Could you check a few things on this model? Use its own coordinates, in mm. Give positions to 0.01 mm unless a question says otherwise; leave off trailing zeros. Loops run counter-clockwise (first coordinate to the right, second up) from the corner with the lowest first, then second, coordinate; pieces in that order, holes last. Notation, with made-up numbers: M 58,-29 L 93,-29 A20 ccw 93,10 Z; hole C 83.25,-13.75 d3. An arc over 180 degrees is marked long. Answer in a Markdown table with one row per item. Add a question column.
1. If we section it at B-B on z = 8: List the corners of the cut face in (x, y) for me.
2. I need wall thicknesses on line 1 along Y through (x, z) = (3.25, -14); line 2 along Y through (x, z) = (1.75, 40); line 3 along Z through (x, y) = (2.5, -50). Which ranges of each line are inside material? Lowest first, please. Write a range as from..to.
3. If we section it at A-A on y = -52: List the corners of the cut face in (x, z) for me, then the cut area to 3 significant figures.
4. If we section it at C-C on y = 33: List the corners of the cut face in (x, z) for me.
5. Thinking about a two-plate mould opening in Z: for faces 1 (the flat face through (10, -1, 1)), 2 (the flat face through (5, 1, 60)), 3 (the flat face through (2, -1, 0)), which applies, released by +Z, released by -Z, zero draft, split by the parting line, or undercut?
6. I'm going to push flat-ended pins straight in: pin 1 Ø8 at (y, z) = (-28, -11) entering from -X; pin 2 Ø1.5 at (y, z) = (61.25, 0) entering from -X. Where does each tip first touch, or does it pass through?
Autodesk Inventor part; units mm, degrees
ref_plane "YZ Plane" through (0, 0, 0) normal (1, 0, 0) x (0, 1, 0)
ref_plane "XZ Plane" through (0, 0, 0) normal (0, 1, 0) x (-1, 0, 0)
ref_plane "XY Plane" through (0, 0, 0) normal (0, 0, 1) x (1, 0, 0)
sketch "Boceto1" plane through (0, 0, 0) normal (1, 0, 0) x (0, 1, 0)
  line L0 (-57.5, -42.7876) -> (57.5, -42.7876)
  line L1 (57.5, -42.7876) -> (57.5, 42.2124)
  line L2 (57.5, 42.2124) -> (-57.5, 42.2124)
  line L3 (-57.5, 42.2124) -> (-57.5, -42.7876)
  line L4 (-57.5, -42.7876) -> (57.5, 42.2124) construction
  line L5 (57.5, -42.7876) -> (-57.5, 42.2124) construction
  point P0 (0, 0)
  point P1 (0, -0.2876)
  dimension "d0" = 115
  dimension "d1" = 85
sketch "Boceto2" plane through (0, 0, 0) normal (1, 0, 0) x (0, 1, 0)
  line L0 (-65, -60) -> (65, -60)
  line L1 (65, -60) -> (65, 60)
  line L2 (65, 60) -> (-65, 60)
  line L3 (-65, 60) -> (-65, -60)
  line L4 (-65, -60) -> (65, 60) construction
  line L5 (65, -60) -> (-65, 60) construction
  point P0 (0, 0)
  dimension "d2" = 130
  dimension "d3" = 120
extrude "Extrusión1" add sketch "Boceto2" along normal blind 10
extrude "Extrusión2" cut sketch "Boceto1" along normal blind 2
sketch "Boceto3" plane through (0, 0, 0) normal (-1, 0, 0) x (0, 0, 1)
  line L0 (0, 0) -> (0, -52)
  line L1 (0, 0) -> (0, 52)
  line L2 (-60, -65) -> (-60, 65)
  line L3 (0, -52) -> (46, -52)
  line L4 (0, -52) -> (-46, -52)
  line L5 (-46, -52) -> (-48.5, -52)
  circle A0 centre (-48.5, -52) radius 2.5
  line L6 (46, -52) -> (48.5, -52)
  circle A1 centre (48.5, -52) radius 2.5
  line L7 (0, 52) -> (48.5, 52)
  line L8 (0, 52) -> (-48.5, 52)
  line L9 (-42.7876, -57.5) -> (-42.7876, 57.5)
  circle A2 centre (-48.5, 52) radius 2.5
  circle A3 centre (48.5, 52) radius 2.5
  dimension "d8" = 52
  dimension "d9" = 52
  dimension "d10" = 46
  dimension "d11" = 46
  dimension "d12" = 2.5
  dimension "d13" = 2.5
  dimension "d14" = 48.5
  dimension "d15" = 5
  dimension "d16" = 5
extrude "Extrusión3" cut sketch "Boceto3" against normal through all contours A1 | A0 | A2 | A3
chamfer "Chaflán1" distance 2.3 angle 45 4 edges at (0, 52, -51) (0, -52, -51) (0, -52, 46) (0, 52, 46)
sketch "Boceto5" plane through (0, 0, 0) normal (-1, 0, 0) x (0, 0, 1)
  circle A0 centre (-48.5, 52) radius 2.5
  circle A1 centre (-48.5, -52) radius 2.5
  line L0 (-48.5, 52) -> (-48.5, -52)
  line L1 (-48.5, 52) -> (-48.5, 44)
  line L2 (-48.5, 52) -> (-48.5, 38)
  circle A2 centre (-48.5, 0) radius 1.25
  circle A3 centre (-48.5, -14) radius 1.25
  circle A4 centre (-48.5, -28) radius 1.25
  circle A5 centre (-48.5, 14) radius 1.25
  circle A6 centre (-48.5, 28) radius 1.25
  circle A7 centre (-48.5, 42) radius 1.25
  line L3 (-48.5, -28) -> (-48.5, -42)
  circle A8 centre (-48.5, -42) radius 1.25
  line L4 (0, 0) -> (0, -23.0144)
  circle A9 centre (48.5, 0) radius 1.25
  circle A10 centre (48.5, -14) radius 1.25
  circle A11 centre (48.5, -28) radius 1.25
  circle A12 centre (48.5, 14) radius 1.25
  circle A13 centre (48.5, 28) radius 1.25
  circle A14 centre (48.5, 42) radius 1.25
  circle A15 centre (48.5, -42) radius 1.25
  dimension "d27" = 2.5
  dimension "d30" = 14
  dimension "d37" = 14
  dimension "d42" = 14
  dimension "d43" = 2.5
extrude "Extrusión4" cut sketch "Boceto5" against normal through all contours A8 L0 | L0 A8 | A4 L0 | L0 A4 | A3 L0 | L0 A3 | A2 L0 | L0 A2 | A5 L0 | L0 A5 | A6 L0 | L0 A6 | A7 L0 | L0 A7 | A9 | A10 | A11 | A12 | A13 | A14 | A15
sketch "Boceto6" plane through (0, 0, 0) normal (-1, 0, 0) x (0, 0, 1)
  line L0 (60, -65) -> (-60, -65)
  line L1 (42.2124, -57.5) -> (-42.7876, -57.5)
  line L2 (0, -57.5) -> (0, -65)
  circle A0 centre (0, -61.25) radius 1.25
  circle A1 centre (-14, -61.25) radius 1.25
  circle A2 centre (-28, -61.25) radius 1.25
  circle A3 centre (14, -61.25) radius 1.25
  circle A4 centre (28, -61.25) radius 1.25
  line L3 (0, 0) -> (18.5256, 0)
  circle A5 centre (0, 61.25) radius 1.25
  circle A6 centre (-14, 61.25) radius 1.25
  circle A7 centre (-28, 61.25) radius 1.25
  circle A8 centre (14, 61.25) radius 1.25
  circle A9 centre (28, 61.25) radius 1.25
  dimension "d46" = 2.5
  dimension "d49" = 14
  dimension "d56" = 14
extrude "Extrusión5" cut sketch "Boceto6" against normal through all
sketch "Boceto7" plane through (0, 0, 0) normal (-1, 0, 0) x (0, 0, 1)
  circle A0 centre (48.5, 42) radius 1.25
  line L0 (48.5, 42) -> (48.5, 39)
  line L1 (48.5, 39) -> (52.5, 39)
  line L2 (52.5, 39) -> (52.5, 45)
  line L3 (52.5, 45) -> (40.5, 45)
  line L4 (40.5, 45) -> (25.5, 45)
  point P0 (0, 0)
  dimension "d63" = 3
  dimension "d64" = 4
  dimension "d65" = 6
  dimension "d66" = 12
  dimension "d67" = 15
properties part number "Soporte PCB"
Results:
| question | item | result |
|---|---|---|
| 1 | outline | M 0,-65 L 10,-65 L 10,65 L 0,65 L 0,57.5 L 2,57.5 L 2,-57.5 L 0,-57.5 Z |
| 2 | line 1 | -65..-62.5, -60..60, 62.5..65 |
| 2 | line 2 | -65..-57.5, 57.5..65 |
| 2 | line 3 | -60..-50, -47..47, 50..60 |
| 3 | outline | M 0,-60 L 10,-60 L 10,-51 L 2.3,-51 L 0,-53.3 Z; M 0,-43.7 L 2.3,-46 L 10,-46 L 10,46 L 2.3,46 L 0,43.7 L 0,42.21 L 2,42.21 L 2,-42.79 L 0,-42.79 Z; M 0,53.3 L 2.3,51 L 10,51 L 10,60 L 0,60 Z |
| 3 | area | 919 mm2 |
| 4 | outline | M 0,-60 L 10,-60 L 10,60 L 0,60 L 0,42.21 L 2,42.21 L 2,-42.79 L 0,-42.79 Z |
| 5 | face 1 | zero draft |
| 5 | face 2 | released by +Z |
| 5 | face 3 | undercut |
| 6 | pin 1 | x = 2 |
| 6 | pin 2 | through |
